Answer from the drawing. Dimensions are ordinates in mm from the lowest x, y and z of the part. Give positions to 0.01 mm unless a question says otherwise; leave off trailing zeros.
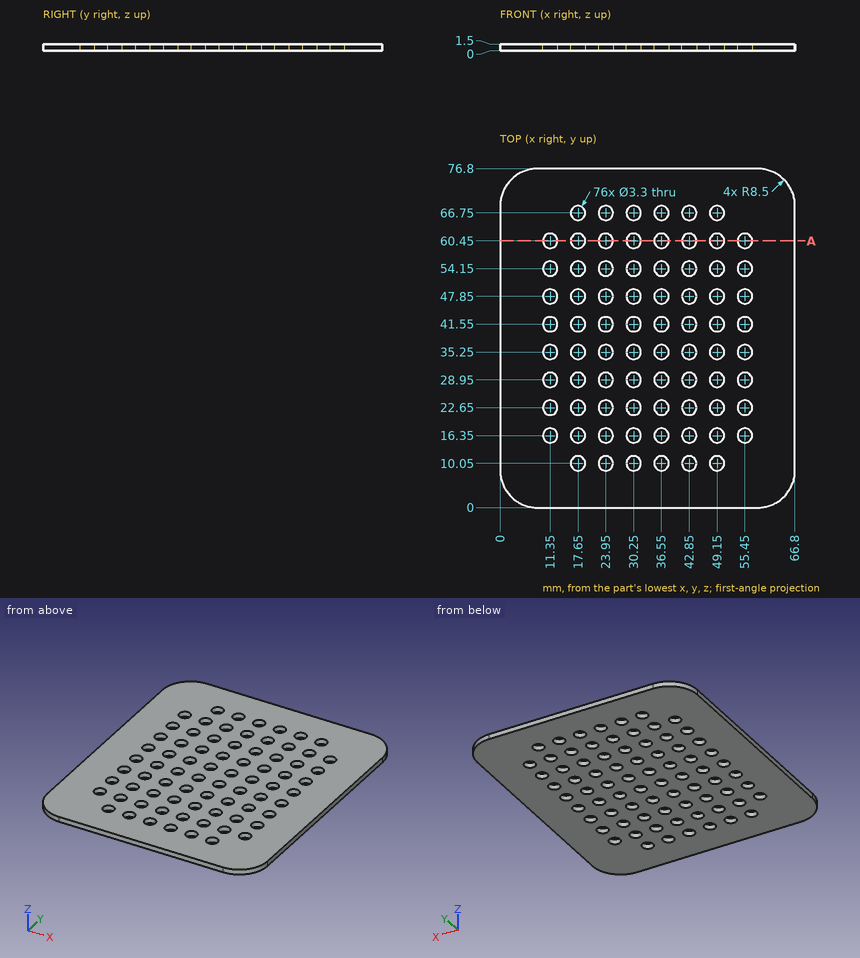
Item 1: This flat-tipped pin is pushed along its axis until it touches: pin 1 Ø2 at (x, y) = (30.25, 54.15) entering from +Z. Where does it stop, or does it pass through?
Result set:
pin 1: passes through
Item 2: Section A-A (y = 60.45) is taken. Give the number of separate pieces and of enclosed holes in the cut face, and give its area (3 significant figures).
Result set:
separate pieces: 9
enclosed holes: 0
area: 60.6 mm2
Item 3: Find the intervals of material crossed by line 1 along X through (y, z) = (8, 1.3), in increasing order.
Result set:
line 1: x = 0.01 to 66.79
